from build123d import *

# Parameters (mm, degrees)
F0_R     = 0.75
F0_W     = 38.1
F0_H     = 3.175
F1_DEPTH = 3.175


with BuildPart() as f1:
    # F0 (on Right) → F1 (new body)
    with BuildSketch(Plane.YZ):
        Polygon((0, 8.73125), (0, 0), (4.7625, 0), (4.7625, 3.175), (4.7625, 14.2875), (4.7625, 17.4625), (2.38125, 17.4625), (0, 17.4625), align=None)
        with Locations((2.38125, 8.73125)):
            Circle(F0_R, mode=Mode.SUBTRACT)
        with Locations((23.8125, 1.5875)):
            Rectangle(F0_W, F0_H)
        with Locations((23.8125, 15.875)):
            Rectangle(F0_W, F0_H)
        Polygon((42.8625, 3.175), (42.8625, 0), (47.625, 0), (47.625, 17.4625), (42.8625, 17.4625), (42.8625, 14.2875), align=None)
        with Locations((45.24375, 8.73125)):
            Circle(F0_R, mode=Mode.SUBTRACT)
    extrude(amount=F1_DEPTH)


solid = f1.part
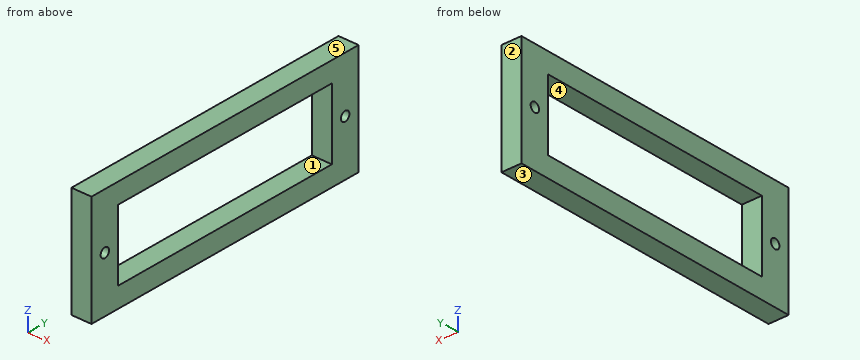
Geometry check sheet. Reference: the model listing, model coordinates, mm. Face numbers are marked on the shaded views. A direction names the side the tool comes from. Give positions to 0.01 mm unless a question says otherwise; leave off trailing zeros. Order: outer loops, then holes, each group sorted by start corner. A loop starts at its lowest first (then second) coordinate and runs counter-clockwise, first axis right, second up. Notation, with made-up numbers: M 62.25,44.25 L 71.25,44.25 A30 ccw 71.25,74.25 Z; hole C -35.75,-23 d11. An arc over 180 degrees is marked long. Use a Markdown table: item, result.
Item 1: Section check B-B (z = 6.5). Record the cut outline in (x, y) (1 decimal), and give its area (3 significant figures).
Answers follow:
| item | result |
|---|---|
| outline | M 0,0 L 3.2,0 L 3.2,4.8 L 0,4.8 Z; M 0,42.9 L 3.2,42.9 L 3.2,47.6 L 0,47.6 Z |
| area | 30.2 mm2 |
Item 2: Section check C-C (x = 1.1). State how many separate pieces and enclosed holes the cut face has, and give its area (3 significant figures).
Answers follow:
| item | result |
|---|---|
| separate pieces | 1 |
| enclosed holes | 3 |
| area | 405 mm2 |
Item 3: Section check A-A (y = 11). Record the cut outline in (x, z) (1 decimal).
Answers follow:
| item | result |
|---|---|
| outline | M 0,0 L 3.2,0 L 3.2,3.2 L 0,3.2 Z; M 0,14.3 L 3.2,14.3 L 3.2,17.5 L 0,17.5 Z |
Item 4: Tool access check on the marked faces 4 and 5. Record the directions out of +Z, -Z, +X, -X, +Y, -Y that give a thin tool (end or side, any length) a straight path to the whole face; none if there is none.
Answers follow:
| item | result |
|---|---|
| face 4 | +X, -X |
| face 5 | +Z, +X, -X, +Y, -Y |
Item 5: Draft check along Z on the marked faces 1, 2 and 3. Enter one of: +Z half, -Z half, draft (parallel to the pull), parting line (faces both ways), or undercut.
Answers follow:
| item | result |
|---|---|
| face 1 | undercut |
| face 2 | draft |
| face 3 | -Z half |
Item 6: Material ranges on line 1 along Z through (x, y) = (1.4, 16) (1 decimal); line 2 along Y through (x, z) = (2.85, 12) (1 decimal), recorded low to high.
Answers follow:
| item | result |
|---|---|
| line 1 | z = 0 to 3.2, 14.3 to 17.5 |
| line 2 | y = 0 to 4.8, 42.9 to 47.6 |
